Source: CAD feature listing. Evaluate the final solid. Frame: model axes, mm. A direction names the side the tool comes from. Round coordinates to 2 decimals unless told otherwise and drop trailing zeros. Loops run counter-clockwise (first coordinate to the right, second up) from the corner with the lowest first, then second, coordinate; pieces in that order, holes last. Notation, with made-up numbers: M -19.75,30.5 L 23.25,30.5 A5 ccw 23.25,36.5 Z; hole C 19,63.25 d11. An arc over 180 degrees is marked long. Answer as a JSON object with one key per item and string values.
from build123d import *

# Parameters (mm, degrees)
BASE_FLANGE1_DEPTH           = 2.05232
EDGE_FLANGE1_STRIP_W         = 9.68248
EDGE_FLANGE1_STRIP_H         = 2.05232
EDGE_FLANGE1_STRIP_CUT_DEPTH = 673.1
EDGE_FLANGE1_DEPTH           = 673.1
SKETCH9_R                    = 3.3782
CUT_EXTRUDE1_DEPTH           = 2.54
SKETCH11_R                   = 2.5
CUT_EXTRUDE2_DEPTH           = 2.54
SKETCH12_R                   = 3.3782
SKETCH12_R_2                 = 14.2875
SKETCH12_R_3                 = 2.0193
CUT_EXTRUDE3_DEPTH           = 2.54
FILLET1_R                    = 2.54
SKETCH13_R                   = 5.5626
SKETCH13_R_2                 = 11.1125
SKETCH13_R_3                 = 14.2875
CUT_EXTRUDE4_DEPTH           = 2.54
SKETCH14_R                   = 3.3782
CUT_EXTRUDE5_DEPTH           = 2.54


# Sheet-metal steps are written as plain solids
with BuildPart() as part:
    # Sketch1 → Base-Flange1 (new body)
    with BuildSketch(Plane.XY):
        with BuildLine():
            Line((-279.272286306, -371.833913043), (-279.272286306, 285.935830835))
            ThreePointArc((-279.272286306, 285.935830835), (-275.352326101, 291.802465867), (-268.432158245, 290.425958896))
            Line((-268.432158245, 290.425958896), (393.827713694, -219.433913043))
            Line((393.827713694, -219.433913043), (393.827713694, -371.833913043))
            Line((393.827713694, -371.833913043), (-279.272286306, -371.833913043))
        make_face()
    extrude(amount=-BASE_FLANGE1_DEPTH)

    # Edge-Flange1 strip (across the edge) → Edge-Flange1 strip cut (cut)
    with BuildSketch(Plane(origin=(-279.272286306, -371.833913043, 0), x_dir=(0, 1, 0), z_dir=(1, 0, 0))):
        with Locations((-2.05232, -1.02616)):
            Rectangle(EDGE_FLANGE1_STRIP_W, EDGE_FLANGE1_STRIP_H)
    extrude(amount=EDGE_FLANGE1_STRIP_CUT_DEPTH, mode=Mode.SUBTRACT)

    # Edge-Flange1 section (across the edge) → Edge-Flange1 (add)
    with BuildSketch(Plane(origin=(-279.272286306, -371.833913043, 0), x_dir=(0, 1, 0), z_dir=(1, 0, 0))):
        with BuildLine():
            Line((0, 0.7366), (0, 83.03768))
            Line((0, 83.03768), (2.05232, 83.03768))
            Line((2.05232, 83.03768), (2.05232, 0.7366))
            ThreePointArc((2.05232, 0.7366), (2.268065145, 0.215745145), (2.78892, 0))
            Line((2.78892, 0), (2.78892, -2.05232))
            ThreePointArc((2.78892, -2.05232), (0.816855756, -1.235464244), (0, 0.7366))
        make_face()
    extrude(amount=EDGE_FLANGE1_DEPTH)

    # Sketch9 → Cut-Extrude1 (cut)
    with BuildSketch(Plane(origin=(0, -369.781593043, 0), x_dir=(1, 0, 0), z_dir=(0, 1, 0))):
        with Locations(Location((381.127713694, -76.68768, 0), (0, 0, 270))):
            Circle(SKETCH9_R)
        with Locations(Location((316.357713694, -76.68768, 0), (0, 0, 270))):
            Circle(SKETCH9_R)
        with Locations(Location((251.587713694, -76.68768, 0), (0, 0, 270))):
            Circle(SKETCH9_R)
        with Locations(Location((186.817713694, -76.68768, 0), (0, 0, 270))):
            Circle(SKETCH9_R)
        with Locations(Location((122.047713694, -76.68768, 0), (0, 0, 270))):
            Circle(SKETCH9_R)
        with Locations(Location((57.277713694, -76.68768, 0), (0, 0, 270))):
            Circle(SKETCH9_R)
        with Locations(Location((-7.492286306, -76.68768, 0), (0, 0, 270))):
            Circle(SKETCH9_R)
        with Locations(Location((-72.262286306, -76.68768, 0), (0, 0, 270))):
            Circle(SKETCH9_R)
        with Locations(Location((-137.032286306, -76.68768, 0), (0, 0, 270))):
            Circle(SKETCH9_R)
        with Locations(Location((-201.802286306, -76.68768, 0), (0, 0, 270))):
            Circle(SKETCH9_R)
        with Locations(Location((-266.572286306, -76.68768, 0), (0, 0, 270))):
            Circle(SKETCH9_R)
        with Locations(Location((368.427713694, -4.29768, 0), (0, 0, 270))):
            Circle(SKETCH9_R)
        with Locations(Location((306.197713694, -4.29768, 0), (0, 0, 270))):
            Circle(SKETCH9_R)
        with Locations(Location((243.967713694, -4.29768, 0), (0, 0, 270))):
            Circle(SKETCH9_R)
        with Locations(Location((181.737713694, -4.29768, 0), (0, 0, 270))):
            Circle(SKETCH9_R)
        with Locations(Location((119.507713694, -4.29768, 0), (0, 0, 270))):
            Circle(SKETCH9_R)
        with Locations(Location((57.277713694, -4.29768, 0), (0, 0, 270))):
            Circle(SKETCH9_R)
        with Locations(Location((-4.952286306, -4.29768, 0), (0, 0, 270))):
            Circle(SKETCH9_R)
        with Locations(Location((-67.182286306, -4.29768, 0), (0, 0, 270))):
            Circle(SKETCH9_R)
        with Locations(Location((-129.412286306, -4.29768, 0), (0, 0, 270))):
            Circle(SKETCH9_R)
        with Locations(Location((-191.642286306, -4.29768, 0), (0, 0, 270))):
            Circle(SKETCH9_R)
        with Locations(Location((-253.872286306, -4.29768, 0), (0, 0, 270))):
            Circle(SKETCH9_R)
    extrude(amount=-CUT_EXTRUDE1_DEPTH, mode=Mode.SUBTRACT)

    # Sketch11 → Cut-Extrude2 (cut)
    with BuildSketch(Plane.XY):
        with Locations((-269.272286306, 260.799452815)):
            Circle(SKETCH11_R)
        with Locations((-269.272286306, 108.399452815)):
            Circle(SKETCH11_R)
        with Locations((-269.272286306, -44.000547185)):
            Circle(SKETCH11_R)
        with Locations((-269.272286306, -196.400547185)):
            Circle(SKETCH11_R)
        with Locations((-269.272286306, -348.800547185)):
            Circle(SKETCH11_R)
        with Locations((-243.872286306, 260.799452815)):
            Circle(SKETCH11_R)
        with Locations((-243.872286306, 108.399452815)):
            Circle(SKETCH11_R)
        with Locations((-243.872286306, -44.000547185)):
            Circle(SKETCH11_R)
        with Locations((-243.872286306, -196.400547185)):
            Circle(SKETCH11_R)
        with Locations((-243.872286306, -348.800547185)):
            Circle(SKETCH11_R)
    extrude(amount=-CUT_EXTRUDE2_DEPTH, mode=Mode.SUBTRACT)

    # Sketch12 → Cut-Extrude3 (cut)
    with BuildSketch(Plane(origin=(0, 0, -2.05232), x_dir=(-1, 0, 0), z_dir=(0, 0, -1))):
        with Locations((-374.777713694, -220.79547031)):
            Circle(SKETCH12_R)
        with Locations((-374.777713694, -331.92047031)):
            Circle(SKETCH12_R)
        with Locations((-263.652713694, -331.92047031)):
            Circle(SKETCH12_R)
        with Locations((-263.652713694, -220.79547031)):
            Circle(SKETCH12_R)
        with Locations((-196.977713694, -168.633913043)):
            Circle(SKETCH12_R_2)
        with Locations((126.872286306, -168.633913043)):
            Circle(SKETCH12_R_2)
        with Locations((-222.165699247, -165.358949868)):
            Circle(SKETCH12_R_3)
        with Locations((-171.789728141, -171.908876219)):
            Circle(SKETCH12_R_3)
    extrude(amount=-CUT_EXTRUDE3_DEPTH, mode=Mode.SUBTRACT)

    # Fillet1
    fillet1_edges = [part.edges().sort_by_distance(p)[0] for p in [
        (393.827713694, -219.433913043, -1.02616),
    ]]
    fillet(fillet1_edges, radius=FILLET1_R)

    # Sketch13 → Cut-Extrude4 (cut)
    with BuildSketch(Plane(origin=(0, 0, -2.05232), x_dir=(-1, 0, 0), z_dir=(0, 0, -1))):
        with Locations((-287.465213694, -314.566215277)):
            Circle(SKETCH13_R)
        with Locations((-312.865213694, -314.566215277)):
            Circle(SKETCH13_R)
        with Locations((-338.265213694, -314.566215277)):
            Circle(SKETCH13_R)
        with Locations((-298.869813694, -276.35797031)):
            Circle(SKETCH13_R_2)
        with Locations((-339.560613694, -276.35797031)):
            Circle(SKETCH13_R_3)
        with Locations((-287.465213694, -238.149725343)):
            Circle(SKETCH13_R)
        with Locations((-312.865213694, -238.149725343)):
            Circle(SKETCH13_R)
        with Locations((-338.265213694, -238.149725343)):
            Circle(SKETCH13_R)
    extrude(amount=-CUT_EXTRUDE4_DEPTH, mode=Mode.SUBTRACT)

    # Sketch14 → Cut-Extrude5 (cut)
    with BuildSketch(Plane.XY):
        with Locations((-226.880308275, 242.408318762)):
            Circle(SKETCH14_R)
        with Locations((-196.690792188, 219.166048683)):
            Circle(SKETCH14_R)
        with Locations((-166.501276101, 195.923778604)):
            Circle(SKETCH14_R)
        with Locations((-136.311760014, 172.681508525)):
            Circle(SKETCH14_R)
        with Locations((-106.122243926, 149.439238446)):
            Circle(SKETCH14_R)
        with Locations((-75.932727839, 126.196968367)):
            Circle(SKETCH14_R)
        with Locations((-45.743211752, 102.954698288)):
            Circle(SKETCH14_R)
        with Locations((-15.553695665, 79.712428209)):
            Circle(SKETCH14_R)
        with Locations((14.635820422, 56.47015813)):
            Circle(SKETCH14_R)
        with Locations((44.825336509, 33.227888051)):
            Circle(SKETCH14_R)
        with Locations((75.014852596, 9.985617972)):
            Circle(SKETCH14_R)
        with Locations((105.204368683, -13.256652107)):
            Circle(SKETCH14_R)
        with Locations((135.393884771, -36.498922186)):
            Circle(SKETCH14_R)
        with Locations((165.583400858, -59.741192265)):
            Circle(SKETCH14_R)
        with Locations((195.772916945, -82.983462344)):
            Circle(SKETCH14_R)
        with Locations((225.962433032, -106.225732423)):
            Circle(SKETCH14_R)
        with Locations((256.151949119, -129.468002502)):
            Circle(SKETCH14_R)
        with Locations((286.341465206, -152.710272581)):
            Circle(SKETCH14_R)
        with Locations((316.530981293, -175.95254266)):
            Circle(SKETCH14_R)
        with Locations((346.720497381, -199.194812739)):
            Circle(SKETCH14_R)
    extrude(amount=-CUT_EXTRUDE5_DEPTH, mode=Mode.SUBTRACT)


solid = part.part
Item 1: Line query: probe 1 along Y at (x, z) = (298.5, 21.5); probe 2 along Z at (x, y) = (-1, -243). Output: solid intervals per line, ascending. Write a range as from..to.
Answer sheet:
{"probe 1": "y = -371.83..-369.78", "probe 2": "z = -2.05..0"}
Item 2: Contact query for flat-ended pins moving along their axis: pin 1 Ø11 at (x, y) = (256.15, -129.47) entering from +Z; pin 2 Ø8 at (x, z) = (-19, 52.5) entering from +Y. Output: stop coordinate, or through.
Answer sheet:
{"pin 1": "stops at z = 0", "pin 2": "stops at y = -369.78"}
Item 3: Section B-B on y = -298.5. Return the cut outline in (x, z).
Answer sheet:
{"outline": "M -279.27,-2.05 L 393.83,-2.05 L 393.83,0 L -279.27,0 Z"}
Item 4: Pull-direction query (X, two-part tool) for faces 1 (the flat face through (53, -371.834, 41)), 2 (the cylindrical face through (-112.6, -168, -1)), 3 (the flat face through (393.828, -295.9, -0.3)), 4 (the cylindrical face through (183.35, -164.34, -1.04)); classes: pulls with the +X half, pulls with the -X half, needs draft (parallel to the pull), parting line crosses it, or undercut.
Answer sheet:
{"face 1": "needs draft", "face 2": "undercut", "face 3": "pulls with the +X half", "face 4": "undercut"}
Item 5: Section A-A on z = 46. Return the cut outline in (x, y), then the cut area to 3 significant figures.
Answer sheet:
{"outline": "M -279.27,-371.83 L 393.83,-371.83 L 393.83,-369.78 L -279.27,-369.78 Z", "area": "1,380 mm²"}
Item 6: Access query for faces 5 (the flat face through (-13, -107, 0)), 6 (the flat face through (-13, -107, -2.052)). Directions: +Z, -Z, +X, -X, +Y, -Y. A direction counts if a zero-diameter tool reaches every point of the face in a straight line with its end or side. Return the directions, or none.
Answer sheet:
{"face 5": "+Z, +X, -X, +Y", "face 6": "-Z, +X, -X, +Y, -Y"}
